Design review of the part built by this model. Coordinates are the model's own, in mm. A direction names the side the tool comes from. Coordinates: 2 decimals unless noted, no trailing zeros. Order: outer loops, then holes, each group sorted by start corner. A loop starts at its lowest first (then second) coordinate and runs counter-clockwise, first axis right, second up. Notation, with made-up numbers: (-21, -11.75) -> (10, -11.75) arc R26 ccw to (10, 15.25) -> close; hole circle Ø5 at (52, 66.5). An arc over 180 degrees is marked (long way). Use a Markdown table: item, result. Add a question column.
Q1. Insertion check: pin 1 (0.5 mm diameter, centred on y = 18.5, z = 4, fed in from +X); pin 2 (5 mm diameter, centred on y = 7.5, z = 4, fed in from -X); pin 3 (3 mm diameter, centred on x = 48, y = 9, fed in from +Z). Each pin has a flat end and moves straight along its axis. Give the tip position at first contact, or say it passes through.
Q2. Machinability: for faces 4 (the face through (53.82, 19.3, 2.29)), 5 (the face through (48, 17.95, 2)), 6 (the face through (27, 4, 8)), which of the approach directions +Z, -Z, +X, -X, +Y, -Y give a long, thin tool a straight path to every point of the face, cutting with its end or side? Answer none if there is none.
Q3. Add section C-C (y = 13.25). State the section outline as (x, z) points.
Q4. Add section A-A (z = 5). Count the separate pieces of the cut face and the enclosed holes in it, then the cut area to 3 significant figures.
Q5. Wall thickness on probe 1 along X at (y, z) = (13.5, 1); probe 2 along X at (y, z) = (9.25, 3); probe 3 along X at (y, z) = (17, 1): over which ranges is each line inside the solid? List them lowest first.
Q6. Add section B-B (x = 6). State the section outline as (y, z) points, then the cut area to 3 significant figures.
Q7. The part is to be moulded in two halves that separate along Y. For faces 1 (the face through (42.3, 4, 5)), 2 (the face through (54.25, 10, 2)), 3 (the face through (0.81, 20.33, 0.64)), say which applies: pulls with the +Y half, pulls with the -Y half, needs draft (parallel to the pull), parting line crosses it, or undercut.
Q8. Add section D-D (z = 0.5). State the section outline as (x, y) points, then the cut area to 3 significant figures.
from build123d import *

# Parameters (mm, degrees)
BOSS_EXTRUDE1_DEPTH = 1.3
BOSS_EXTRUDE3_DEPTH = 3
CUT_EXTRUDE1_DEPTH  = 3
SKETCH11_W          = 6.5
SKETCH11_H          = 9
CUT_EXTRUDE2_DEPTH  = 4.3
SKETCH12_W          = 12.1
SKETCH12_H          = 12.1
CUT_EXTRUDE4_DEPTH  = 1.3
SKETCH17_W          = 14.5
SKETCH17_H          = 14.1
SKETCH17_W_2        = 12.1
SKETCH17_H_2        = 12.1
BOSS_EXTRUDE4_DEPTH = 6.25
CUT_EXTRUDE5_DEPTH  = 4.3
BOSS_EXTRUDE5_DEPTH = 6.25
CUT_EXTRUDE6_START  = -3
CUT_EXTRUDE6_DEPTH  = 23
SKETCH21_W          = 2.5
SKETCH21_H          = 2.5
CUT_EXTRUDE7_DEPTH  = 10
BOSS_EXTRUDE7_DEPTH = 7.6
SKETCH25_W          = 2
SKETCH25_H          = 2
BOSS_EXTRUDE8_DEPTH = 7.6
SKETCH27_W          = 1
SKETCH27_H          = 18.4
CUT_EXTRUDE8_DEPTH  = 7.5


with BuildPart() as part:
    # Sketch1 → Boss-Extrude1 (new body)
    with BuildSketch(Plane.XY):
        with BuildLine():
            Line((2.7, 0), (52.9, 0))
            ThreePointArc((52.9, 0), (54.809188309, 0.790811691), (55.6, 2.7))
            Line((55.6, 2.7), (55.6, 18.4))
            ThreePointArc((55.6, 18.4), (54.809188309, 20.309188309), (52.9, 21.1))
            Line((52.9, 21.1), (2.7, 21.1))
            ThreePointArc((2.7, 21.1), (0.790811691, 20.309188309), (0, 18.4))
            Line((0, 18.4), (0, 2.7))
            ThreePointArc((0, 2.7), (0.790811691, 0.790811691), (2.7, 0))
        make_face()
    extrude(amount=BOSS_EXTRUDE1_DEPTH)

    # Sketch4 → Boss-Extrude3 (add)
    with BuildSketch(Plane.XY.offset(1.3)):
        with BuildLine():
            Line((54.25, 2.85), (54.25, 18.25))
            ThreePointArc((54.25, 18.25), (53.810660172, 19.310660172), (52.75, 19.75))
            Line((52.75, 19.75), (2.85, 19.75))
            ThreePointArc((2.85, 19.75), (1.789339828, 19.310660172), (1.35, 18.25))
            Line((1.35, 18.25), (1.35, 2.85))
            ThreePointArc((1.35, 2.85), (1.789339828, 1.789339828), (2.85, 1.35))
            Line((2.85, 1.35), (52.75, 1.35))
            ThreePointArc((52.75, 1.35), (53.810660172, 1.789339828), (54.25, 2.85))
        make_face()
    extrude(amount=BOSS_EXTRUDE3_DEPTH)

    # Sketch5 → Cut-Extrude1 (cut)
    with BuildSketch(Plane.XY.offset(4.3)):
        with BuildLine():
            Line((51.95, 17.95), (3.65, 17.95))
            ThreePointArc((3.65, 17.95), (3.296446609, 17.803553391), (3.15, 17.45))
            Line((3.15, 17.45), (3.15, 3.65))
            ThreePointArc((3.15, 3.65), (3.296446609, 3.296446609), (3.65, 3.15))
            Line((3.65, 3.15), (51.95, 3.15))
            ThreePointArc((51.95, 3.15), (52.303553391, 3.296446609), (52.45, 3.65))
            Line((52.45, 3.65), (52.45, 17.45))
            ThreePointArc((52.45, 17.45), (52.303553391, 17.803553391), (51.95, 17.95))
        make_face()
    extrude(amount=-CUT_EXTRUDE1_DEPTH, mode=Mode.SUBTRACT)

    # Sketch10 → Cut-Revolve1 (revolve, cut)
    with BuildSketch(Plane(origin=(0, 19.75, 0), x_dir=(1, 0, 0), z_dir=(0, 1, 0))):
        with BuildLine():
            Line((41.7, -2), (41.7, -3.6))
            ThreePointArc((41.7, -3.6), (40.9, -2.8), (41.7, -2))
        make_face()
    cut_revolve1 = revolve(axis=Axis((41.7, 19.75, 2), (0, 0, 1)), mode=Mode.SUBTRACT)

    # Mirror1: Cut-Revolve1 across plane
    add(cut_revolve1.mirror(Plane(origin=(0, 10.55, 0), x_dir=(0, 0, 1), z_dir=(0, -1, 0))), mode=Mode.SUBTRACT)

    # Sketch11 → Cut-Extrude2 (cut)
    with BuildSketch(Plane(origin=(0, 0, 0), x_dir=(-1, 0, 0), z_dir=(0, 0, -1))):
        with Locations((-5.7, 7)):
            Rectangle(SKETCH11_W, SKETCH11_H)
    extrude(amount=-CUT_EXTRUDE2_DEPTH, mode=Mode.SUBTRACT)

    # Sketch12 → Cut-Extrude4 (cut)
    with BuildSketch(Plane(origin=(0, 0, 0), x_dir=(-1, 0, 0), z_dir=(0, 0, -1))):
        with Locations((-19.75, 10.1)):
            Rectangle(SKETCH12_W, SKETCH12_H)
    extrude(amount=-CUT_EXTRUDE4_DEPTH, mode=Mode.SUBTRACT)

    # Sketch17 → Boss-Extrude4 (add)
    with BuildSketch(Plane(origin=(0, 0, 0), x_dir=(-1, 0, 0), z_dir=(0, 0, -1))):
        with Locations((-19.75, 10.1)):
            Rectangle(SKETCH17_W, SKETCH17_H)
        with Locations((-19.75, 10.1)):
            Rectangle(SKETCH17_W_2, SKETCH17_H_2, mode=Mode.SUBTRACT)
    extrude(amount=-BOSS_EXTRUDE4_DEPTH)

    # Sketch13 → Cut-Extrude5 (cut)
    with BuildSketch(Plane(origin=(0, 0, 0), x_dir=(-1, 0, 0), z_dir=(0, 0, -1))):
        Polygon((-45.055992052, 10.55), (-36.5, 1.994007948), (-27.944007948, 10.55), (-36.5, 19.105992052), align=None)
    extrude(amount=-CUT_EXTRUDE5_DEPTH, mode=Mode.SUBTRACT)

    # Sketch18 → Boss-Extrude5 (add)
    with BuildSketch(Plane(origin=(0, 0, 0), x_dir=(-1, 0, 0), z_dir=(0, 0, -1))):
        Polygon((-46.753048327, 10.55), (-36.5, 0.296951673), (-26.246951673, 10.55), (-36.5, 20.803048327), align=None)
        Polygon((-36.5, 19.105992052), (-45.055992052, 10.55), (-36.5, 1.994007948), (-27.944007948, 10.55), align=None, mode=Mode.SUBTRACT)
    extrude(amount=-BOSS_EXTRUDE5_DEPTH)

    # Sketch20 → Cut-Extrude6 (cut)
    with BuildSketch(Plane.XY.offset(4.3).offset(CUT_EXTRUDE6_START)):
        Polygon((35.446951673, 19.75), (37.553048327, 19.75), (36.5, 20.803048327), align=None)
    cut_extrude6 = extrude(amount=CUT_EXTRUDE6_DEPTH, mode=Mode.SUBTRACT)

    # Mirror2: Cut-Extrude6 across plane
    add(cut_extrude6.mirror(Plane(origin=(0, 10.55, 0), x_dir=(0, 0, 1), z_dir=(0, -1, 0))), mode=Mode.SUBTRACT)

    # Sketch21 → Cut-Extrude7 (cut)
    with BuildSketch(Plane(origin=(0, 0, 0), x_dir=(-1, 0, 0), z_dir=(0, 0, -1))):
        with Locations((-29, 16.6)):
            Rectangle(SKETCH21_W, SKETCH21_H)
    extrude(amount=-CUT_EXTRUDE7_DEPTH, mode=Mode.SUBTRACT)

    # Mirror3: Cut-Revolve1 across plane
    add(cut_revolve1.mirror(Plane.ZY.offset(-27.8)), mode=Mode.SUBTRACT)

    # Mirror3 copy 1 sketch → Mirror3 copy 1 (revolve, cut)
    with BuildSketch(Plane(origin=(55.6, 1.35, 0), x_dir=(-1, 0, 0), z_dir=(0, -1, 0))):
        with BuildLine():
            Line((41.7, -2), (41.7, -3.6))
            ThreePointArc((41.7, -3.6), (40.9, -2.8), (41.7, -2))
        make_face()
    revolve(axis=Axis((13.9, 1.35, 2), (0, 0, 1)), mode=Mode.SUBTRACT)

    # Sketch24 → Boss-Extrude7 (add)
    with BuildSketch(Plane.XY.offset(1.3)):
        Polygon((33.646951673, 3.15), (27, 3.15), (27, 5.65), (31.146951673, 5.65), align=None)
    extrude(amount=BOSS_EXTRUDE7_DEPTH)

    # Sketch25 → Boss-Extrude8 (add)
    with BuildSketch(Plane.XY.offset(1.3)):
        with Locations((43.3, 4.15)):
            Rectangle(SKETCH25_W, SKETCH25_H)
    boss_extrude8 = extrude(amount=BOSS_EXTRUDE8_DEPTH)

    # Mirror4: Boss-Extrude8 across plane
    add(boss_extrude8.mirror(Plane(origin=(0, 10.55, 0), x_dir=(0, 0, 1), z_dir=(0, -1, 0))))

    # Sketch27 → Cut-Extrude8 (cut)
    with BuildSketch(Plane(origin=(54.25, 0, 0), x_dir=(0, 0, -1), z_dir=(1, 0, 0))):
        with Locations((-3.8, 10.55)):
            Rectangle(SKETCH27_W, SKETCH27_H)
    extrude(amount=-CUT_EXTRUDE8_DEPTH, mode=Mode.SUBTRACT)


solid = part.part
Established:
| question | item | result |
|---|---|---|
| 1 | pin 1 | x = 46.75 |
| 1 | pin 2 | x = 1.35 |
| 1 | pin 3 | z = 1.3 |
| 2 | face 4 | +Z, +X, +Y |
| 2 | face 5 | +Z |
| 2 | face 6 | +Z, -X, +Y, -Y |
| 3 | outline | (0, 0) -> (13.7, 0) -> (13.7, 6.25) -> (12.5, 6.25) -> (12.5, 1.3) -> (3.15, 1.3) -> (3.15, 4.3) -> (1.35, 4.3) -> (1.35, 1.3) -> (0, 1.3) -> close; (25.8, 0) -> (30.64, 0) -> (30.64, 6.25) -> (28.95, 6.25) -> (28.95, 1.3) -> (27, 1.3) -> (27, 6.25) -> (25.8, 6.25) -> close; (42.36, 0) -> (55.6, 0) -> (55.6, 1.3) -> (54.25, 1.3) -> (54.25, 3.3) -> (52.45, 3.3) -> (52.45, 1.3) -> (44.05, 1.3) -> (44.05, 6.25) -> (42.36, 6.25) -> close |
| 4 | separate pieces | 3 |
| 4 | enclosed holes | 3 |
| 4 | area | 141 mm^2 |
| 5 | probe 1 | 0 to 13.7, 25.8 to 30.89, 42.11 to 55.6 |
| 5 | probe 2 | 1.35 to 2.45, 12.5 to 13.7, 25.8 to 27, 27.55 to 29.24, 43.76 to 45.45, 52.45 to 54.25 |
| 5 | probe 3 | 0 to 27.75, 30.25 to 34.39, 38.61 to 55.6 |
| 6 | outline | (0, 0) -> (2.5, 0) -> (2.5, 4.3) -> (1.35, 4.3) -> (1.35, 1.3) -> (0, 1.3) -> close; (11.5, 0) -> (21.1, 0) -> (21.1, 1.3) -> (19.75, 1.3) -> (19.75, 4.3) -> (17.95, 4.3) -> (17.95, 1.3) -> (11.5, 1.3) -> close |
| 6 | area | 24.6 mm^2 |
| 7 | face 1 | undercut |
| 7 | face 2 | needs draft |
| 7 | face 3 | pulls with the +Y half |
| 8 | outline | (0, 2.7) arc R2.7 ccw to (2.7, 0) -> (52.9, 0) arc R2.7 ccw to (55.6, 2.7) -> (55.6, 18.4) arc R2.7 ccw to (52.9, 21.1) -> (2.7, 21.1) arc R2.7 ccw to (0, 18.4) -> close; hole (2.45, 2.5) -> (8.95, 2.5) -> (8.95, 11.5) -> (2.45, 11.5) -> close; hole (13.7, 4.05) -> (25.8, 4.05) -> (25.8, 16.15) -> (13.7, 16.15) -> close; hole (27.75, 15.35) -> (30.25, 15.35) -> (30.25, 17.85) -> (27.75, 17.85) -> close; hole (27.94, 10.55) -> (36.5, 1.99) -> (45.06, 10.55) -> (36.5, 19.11) -> close |
| 8 | area | 809 mm^2 |
